Check sheet for the modelled part. Datum: model origin and axes. Units: mm. Face numbers are marked on the shaded views. A direction names the side the tool comes from. Give positions to 0.01 mm unless a question says otherwise; leave off trailing zeros. Order: outer loops, then holes, each group sorted by start corner. A loop starts at its lowest first (then second) coordinate and runs counter-clockwise, first axis right, second up. Notation, with made-up numbers: (-31, 53) -> (-22, 53) arc R24 ccw to (-22, 73) -> close; hole circle Ø8 at (-13.75, -7.75). An arc over 180 degrees is marked (long way). Answer in a Markdown table with one row per item. Add a question column.
(1) Thickness scan on L1, parallel to X at y = 13.5, z = 0 (3 decimals); L2, parallel to Y at x = 25, z = -15. Record the ranges inside material, lowest first. Write a range as [from, to].
(2) Cross-section at B-B (y = 5.5). State how many separate pieces and enclosed holes the cut face has, then the cut area to 3 significant figures.
(3) Release check for a two-part mould opening along Y. For the marked faces 4, 5, 6 and 7 record: released by +Y, released by -Y, zero draft, split by the parting line, or undercut.
(4) Go/stop test with flat-tipped pins: pin 1 (5 mm diameter, centred on x = -8, y = 53, fed in from -Z); pin 2 (2.5 mm diameter, centred on x = 1, z = 18.5, fed in from +Y); pin 3 (2.5 mm diameter, centred on x = 17.5, z = -2, fed in from +Y). Record where each tip stops, or that it passes through.
(5) Set-up check for the marked faces 1, 2 and 3: record each of +Z, -Z, +X, -X, +Y, -Y from which the full face is reachable in a straight line by a thin tool's end or side.
(6) Cross-section at D-D (x = 7). Record the cut outline in (y, z), then the cut area to 3 significant figures.
(7) Cross-section at A-A (z = 0). Record the cut outline in (x, y) (3 decimals), then the cut area to 3 significant figures.
(8) Cross-section at C-C (y = 38). Record the cut outline in (x, z) (3 decimals), then the cut area to 3 significant figures.
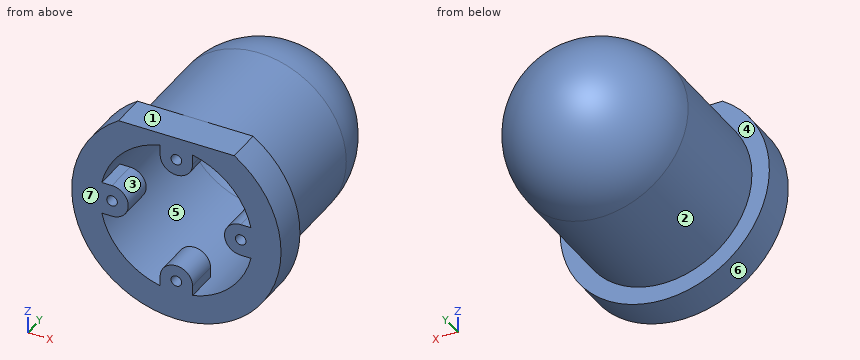
Autodesk Inventor part; units mm, degrees
ref_plane "YZ Plane" through (0, 0, 0) normal (1, 0, 0) x (0, 1, 0)
ref_plane "XZ Plane" through (0, 0, 0) normal (0, 1, 0) x (-1, 0, 0)
ref_plane "XY Plane" through (0, 0, 0) normal (0, 0, 1) x (1, 0, 0)
sketch "Sketch1" plane through (0, 0, 0) normal (0, 0, 1) x (1, 0, 0)
  line L0 (22.225, 0) -> (30.48, 0)
  line L1 (30.48, 0) -> (30.48, 10.16)
  line L2 (30.48, 10.16) -> (25.4, 10.16)
  line L3 (25.4, 10.16) -> (25.4, 44.45)
  line L4 (25.4, 44.45) -> (0, 44.45) construction
  line L5 (0, 10.16) -> (0, 0)
  arc A0 (25.4, 44.45) -> (0, 69.85) centre (0, 44.45) ccw
  line L6 (0, 66.675) -> (0, 69.85)
  arc A1 (22.225, 44.45) -> (0, 66.675) centre (0, 44.45) ccw
  line L7 (22.225, 44.45) -> (22.225, 0)
  line L8 (0, 66.675) -> (0, 0) construction
  line L9 (0, 0) -> (22.225, 0) construction
  dimension "d2" = 3.175
  dimension "d3" = 10.16
  dimension "d4" = 69.85
  dimension "d6" = 25.4
  dimension "d7" = 5.08
revolve "Revolution1" add sketch "Sketch1" angle 360 about axis through (0, 66.675, 0) along (0, -1, 0)
sketch "Sketch3" plane through (0, 0, 0) normal (0, -1, 0) x (1, 0, 0)
  circle A0 centre (0, 0) radius 25.4 construction
  circle A1 centre (0, 0) radius 30.48
  line L0 (0, 25.4) -> (-16.8485, 25.4)
  line L1 (0, 25.4) -> (16.8485, 25.4)
  arc A2 (-16.8485, 25.4) -> (0, 30.48) centre (0, 0) ccw
extrude "Extrusion1" cut sketch "Sketch3" against normal up to next contours L1 L0 A1 picked at (-9.4832, 26.3286)
sketch "Sketch4" plane through (0, 0, 0) normal (0, -1, 0) x (1, 0, 0)
  arc A0 (-18.7397, -4.725) -> (-18.7397, 4.725) centre (-18.7397, 0) ccw
  circle A1 centre (-18.7397, 0) radius 1.55
  line L0 (-18.7397, 4.725) -> (-21.7169, 4.725)
  line L1 (-18.7397, -4.725) -> (-21.7169, -4.725)
  arc A2 (-21.7169, 4.725) -> (-21.7169, -4.725) centre (0, 0) ccw
  point P0 (0, 0)
  dimension "d13" = 3.1
  dimension "d14" = 3.175
extrude "Extrusion2" add sketch "Sketch4" against normal blind 9.652
pattern_circular "Circular Pattern1" count 4 over 360 about axis through (0, 27.305, 0) along (0, -1, 0) of "Extrusion2"
properties part number "led"
Answer below:
| question | item | result |
|---|---|---|
| 1 | L1 | x = [-25.4, -22.225], [22.225, 25.4] |
| 1 | L2 | y = [0, 10.16] |
| 2 | separate pieces | 1 |
| 2 | enclosed holes | 5 |
| 2 | area | 1,490 mm² |
| 3 | face 4 | released by +Y |
| 3 | face 5 | undercut |
| 3 | face 6 | zero draft |
| 3 | face 7 | released by -Y |
| 4 | pin 1 | stops at z = -23.67 |
| 4 | pin 2 | stops at y = 63.07 |
| 4 | pin 3 | stops at y = 63.88 |
| 5 | face 1 | +Z, +X, -X, +Y, -Y |
| 5 | face 2 | +Y |
| 5 | face 3 | -Y |
| 6 | outline | (0, -29.67) -> (10.16, -29.67) -> (10.16, -24.42) -> (44.45, -24.42) arc R24.42 ccw to (44.45, 24.42) -> (10.16, 24.42) -> (10.16, 25.4) -> (0, 25.4) -> (0, 21.09) -> (44.45, 21.09) arc R21.09 cw to (44.45, -21.09) -> (0, -21.09) -> close |
| 6 | area | 596 mm² |
| 7 | outline | (-30.48, 0) -> (-20.29, 0) -> (-20.29, 9.652) -> (-22.225, 9.652) -> (-22.225, 44.45) arc R22.225 cw to (22.225, 44.45) -> (22.225, 9.652) -> (20.29, 9.652) -> (20.29, 0) -> (30.48, 0) -> (30.48, 10.16) -> (25.4, 10.16) -> (25.4, 44.45) arc R25.4 ccw to (-25.4, 44.45) -> (-25.4, 10.16) -> (-30.48, 10.16) -> close; (-17.19, 0) -> (-14.015, 0) -> (-14.015, 9.652) -> (-17.19, 9.652) -> close; (14.015, 0) -> (17.19, 0) -> (17.19, 9.652) -> (14.015, 9.652) -> close |
| 7 | area | 722 mm² |
| 8 | outline | circle Ø50.8 at (0, 0); hole circle Ø44.45 at (0, 0) |
| 8 | area | 475 mm² |
